from build123d import *

# Parameters (mm, degrees)
F0_R     = 3.5
F1_DEPTH = 0.5
F2_R     = 1.9
F2_R_2   = 1.4
F3_DEPTH = 5
F4_W     = 1
F4_H     = 6.460969
F5_DEPTH = 5


with BuildPart() as f1:
    # F0 (on Top) → F1 (new body, symmetric)
    with BuildSketch(Plane.XY):
        Circle(F0_R)
    extrude(amount=F1_DEPTH, both=True)

    # F2 (on face) → F3 (join)
    with BuildSketch(Plane.XY.offset(0.5)):
        Circle(F2_R)
        Circle(F2_R_2, mode=Mode.SUBTRACT)
    extrude(amount=F3_DEPTH)

    # F4 (on face) → F5 (cut)
    with BuildSketch(Plane.XY.offset(5.5)):
        with Locations((0, -0.287181)):
            Rectangle(F4_W, F4_H)
    extrude(amount=-F5_DEPTH, mode=Mode.SUBTRACT)


solid = f1.part
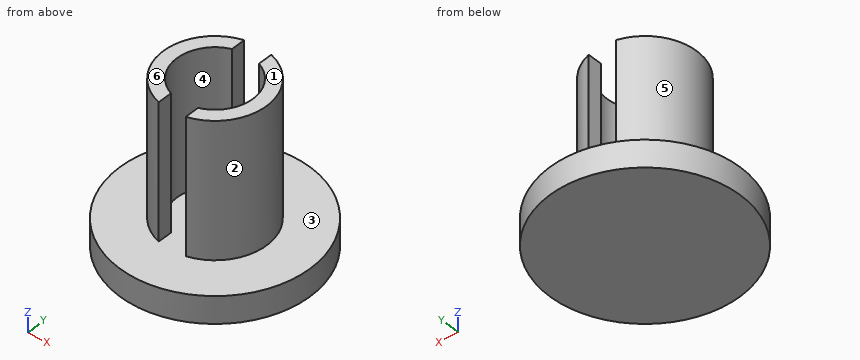
Design review of the part built by this model. Coordinates are the model's own, in mm. Face numbers are marked on the shaded views. A direction names the side the tool comes from. Round coordinates to 2 decimals unless told otherwise and drop trailing zeros. Write each loop counter-clockwise with the first axis right and the second up, starting at its lowest first coordinate (ties: lowest second). Pieces come first, ordered by that corner, then holes.
Item 1: For pin 1 Ø1 at (x, y) = (2.5, 2) entering from +Z; pin 2 Ø0.6 at (y, z) = (1.5, 4) entering from -X; pin 3 Ø2 at (x, z) = (0.5, 2.5) entering from +Y, all flat-tipped, find the tip position at first contact; note any pin that passes through.
Item 2: Consider section C-C on x = 0. Give the boundary of the cut face in (y, z).
Item 3: Draft analysis for pull direction X (two halves, no side actions). For the marked faces 3, 4, 5 and 6, state which applies: released by +X, released by -X, zero draft, split by the parting line, or undercut.
Item 4: Consider section A-A on z = 5.1. Give the boundary of the cut face in (x, y), and give its area (3 significant figures).
Item 5: Wall thickness on L1, parallel to X at y = 0, z = 1.45; L2, parallel to Z at x = 0.75, y = -2; L3, parallel to X at y = 0.5, z = 2.3: over which ranges is each line inside the solid? List them lowest first.
Item 6: For the marked faces 1 and 2, list the 3-axis set-ups (+Z, -Z, +X, -X, +Y, -Y) from which the entire face can be reached by the end or side of a thin tool; tool diameter is ignored.
Item 7: Consider section B-B on y = 0. Give the boundary of the cut face in (x, z).
Item 8: Consider section D-D on y = 0.75. Give the boundary of the cut face in (x, z), and give its area (3 significant figures).
Check values:
1. pin 1: stops at z = 0.5
1. pin 2: stops at x = -1.47
1. pin 3: stops at y = 1.83
2. outline: (-3.5, -0.5) - (3.5, -0.5) - (3.5, 0.5) - (-3.5, 0.5) - close
3. face 3: undercut
3. face 4: undercut
3. face 5: released by -X
3. face 6: zero draft
4. outline: (-0.5, -1.83) - (-0.5, -1.31) arc R1.4 cw to (-0.5, 1.31) - (-0.5, 1.83) arc R1.9 ccw to start; (0.5, -1.83) arc R1.9 ccw to (0.5, 1.83) - (0.5, 1.31) arc R1.4 cw to (0.5, -1.31) - close
4. area: 4.17 mm2
5. L1: x = -1.9 to -1.4, 1.4 to 1.9
5. L2: z = -0.5 to 0.5
5. L3: x = -1.83 to -1.31, 1.31 to 1.83
6. face 1: +Z, +X, -X, +Y, -Y
6. face 2: +Z, +X
7. outline: (-3.5, -0.5) - (3.5, -0.5) - (3.5, 0.5) - (1.9, 0.5) - (1.9, 5.5) - (1.4, 5.5) - (1.4, 0.5) - (-1.4, 0.5) - (-1.4, 5.5) - (-1.9, 5.5) - (-1.9, 0.5) - (-3.5, 0.5) - close
8. outline: (-3.42, -0.5) - (3.42, -0.5) - (3.42, 0.5) - (1.75, 0.5) - (1.75, 5.5) - (1.18, 5.5) - (1.18, 0.5) - (-1.18, 0.5) - (-1.18, 5.5) - (-1.75, 5.5) - (-1.75, 0.5) - (-3.42, 0.5) - close
8. area: 12.5 mm2
